For this review, take the finished solid that the model builds, in its own axes (mm). Face numbers are marked on the shaded views. Coordinates: 2 decimals unless noted, no trailing zeros. Loops run counter-clockwise (first coordinate to the right, second up) from the corner with the lowest first, then second, coordinate; pieces in that order, holes last. Notation, with made-up numbers: M 80,60 L 89,60 A16 ccw 89,83 Z; hole C 13,5.25 d5. An arc over 180 degrees is marked long. Answer as a JSON object with one key per item and string values. Group by question number.
Item 1: Insertion check: pin 1 (1 mm diameter, centred on y = 13.5, z = 1, fed in from +X). The pin has a flat end and moves straight along its axis. Give the tip position at first contact, or say it passes through.
Item 2: Add section B-B (x = 0.45). State the section outline as (y, z) points.
Item 3: Mouldability with a two-part tool opening along Z and no side actions: class the marked faces 1, 2, 3 and 4 as +Z half, -Z half, draft (parallel to the pull), parting line (faces both ways), or undercut.
Item 4: Wall thickness on L1, parallel to Y at x = -0.8, z = -0.6; L2, parallel to X at y = 3, z = 1.25; L3, parallel to X at y = 4, z = 1.65: over which ranges is each line inside the solid? List them lowest first. Write a range as from..to.
Item 5: Add section C-C (y = 10). State the section outline as (x, z) points.
Item 6: Add section A-A (z = 0.15). State the section outline as (x, y) points.
from build123d import *

# Parameters (mm, degrees)
SKETCH1_W           = 3.9
SKETCH1_H           = 3.9
BOSS_EXTRUDE1_DEPTH = 15.5
SKETCH3_W           = 2
SKETCH3_H           = 14
CUT_EXTRUDE1_DEPTH  = 1.707106781
SKETCH4_W           = 3.4
SKETCH4_H           = 3.4
CUT_EXTRUDE2_DEPTH  = 0.25
CUT_EXTRUDE3_DEPTH  = 0.25
CHAMFER1_SIZE       = 1
FILLET1_R           = 0.5


with BuildPart() as part:
    # Sketch1 → Boss-Extrude1 (new body)
    with BuildSketch(Plane(origin=(0, 0, 0), x_dir=(1, 0, 0), z_dir=(0, 1, 0))):
        Rectangle(SKETCH1_W, SKETCH1_H)
    extrude(amount=BOSS_EXTRUDE1_DEPTH)

    # Sketch3 → Cut-Extrude1 (cut, through all)
    with BuildSketch(Plane(origin=(1.45, 0, 1.45), x_dir=(0.707106781, 0, -0.707106781), z_dir=(0.707106781, 0, 0.707106781))):
        with Locations((0, 8.5)):
            Rectangle(SKETCH3_W, SKETCH3_H)
    extrude(amount=CUT_EXTRUDE1_DEPTH, mode=Mode.SUBTRACT)

    # Sketch4 → Cut-Extrude2 (cut)
    with BuildSketch(Plane.XZ):
        Rectangle(SKETCH4_W, SKETCH4_H)
    extrude(amount=-CUT_EXTRUDE2_DEPTH, mode=Mode.SUBTRACT)

    # Sketch5 → Cut-Extrude3 (cut)
    with BuildSketch(Plane.XZ):
        Polygon((1.95, 1.95), (0.85, 1.95), (1.95, 0.85), align=None)
        Polygon((1.95, -1.95), (1.95, -0.85), (0.85, -1.95), align=None)
        Polygon((-1.95, 1.95), (-0.85, 1.95), (-1.95, 0.85), align=None)
        Polygon((-1.95, -1.95), (-0.85, -1.95), (-1.95, -0.85), align=None)
    extrude(amount=-CUT_EXTRUDE3_DEPTH, mode=Mode.SUBTRACT)

    # Chamfer1
    chamfer1_edges = [part.edges().sort_by_distance(p)[0] for p in [
        (1.45, 15.5, 1.45),
    ]]
    chamfer(chamfer1_edges, length=CHAMFER1_SIZE)

    # Fillet1
    fillet1_edges = [part.edges().sort_by_distance(p)[0] for p in [
        (1.45, 1.5, 1.45),
    ]]
    fillet(fillet1_edges, radius=FILLET1_R)


solid = part.part
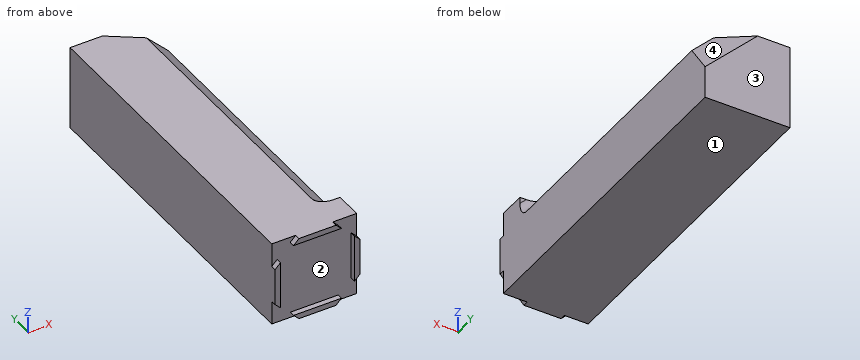
From the geometry:
{
 "1": {"pin 1": "stops at x = 1.95"},
 "2": {"outline": "M 0,-1.95 L 15.5,-1.95 L 15.5,1.04 L 14.85,1.95 L 0,1.95 L 0,1.7 L 0.25,1.7 L 0.25,-1.7 L 0,-1.7 Z"},
 "3": {"face 1": "-Z half", "face 2": "undercut", "face 3": "draft", "face 4": "+Z half"},
 "4": {"L1": "y = 0.25..15.5", "L2": "x = -1.95..1.65", "L3": "x = -1.95..1.25"},
 "5": {"outline": "M -1.95,-1.95 L 1.95,-1.95 L 1.95,0.95 L 0.95,1.95 L -1.95,1.95 Z"},
 "6": {"outline": "M -1.95,0 L -1.7,0 L -1.7,0.25 L 1.7,0.25 L 1.7,0 L 1.95,0 L 1.95,15.07 L 1.34,15.5 L -1.95,15.5 Z"}
}
